from build123d import *

# Parameters (mm, degrees)
ESQUISSE2_W = 4
ESQUISSE2_H = 26
CONG_2_R    = 1
ESQUISSE3_W = 1.417366919
ESQUISSE3_H = 0.8


with BuildPart() as part:
    # Esquisse2 → Révolution1 (revolve)
    with BuildSketch(Plane.XY, mode=Mode.PRIVATE) as r_volution1_sk:
        with Locations((2, 13)):
            Rectangle(ESQUISSE2_W, ESQUISSE2_H)
    revolve(r_volution1_sk.sketch.rotate(Axis((0, 0, 0), (0, 1, 0)), 90), axis=Axis((0, 0, 0), (0, 1, 0)))

    # Congé2
    cong_2_edges = [part.edges().sort_by_distance(p)[0] for p in [
        (0, 0, 4),
        (0, 26, 4),
    ]]
    fillet(cong_2_edges, radius=CONG_2_R)

    # Esquisse3 → Enlèvement de matière-Révolution1 (revolve, cut)
    with BuildSketch(Plane.XY, mode=Mode.PRIVATE) as enl_vement_de_mati_re_r_volution1_sk:
        with Locations((-3.731857201, 21.6)):
            Rectangle(ESQUISSE3_W, ESQUISSE3_H)
    revolve(enl_vement_de_mati_re_r_volution1_sk.sketch.rotate(Axis((0, 0, 0), (0, -1, 0)), 270), axis=Axis((0, 0, 0), (0, -1, 0)), mode=Mode.SUBTRACT)


solid = part.part
For this review, take the finished solid that the model builds, in its own axes (mm). A direction names the side the tool comes from. Give positions to 0.01 mm unless a question says otherwise; leave off trailing zeros. Loops run counter-clockwise (first coordinate to the right, second up) from the corner with the lowest first, then second, coordinate; pieces in that order, holes last. Notation, with made-up numbers: (13.25, -9.75) -> (61.25, -9.75) arc R25 cw to (61.25, 29.25) -> close; hole circle Ø4 at (42.25, -32.5). An arc over 180 degrees is marked (long way). One line per question, with ' | ' between items.
1) Insertion check: pin 1 Ø4 at (x, y) = (-2.5, 4) entering from +Z; pin 2 Ø3 at (y, z) = (20, 2) entering from +X. Each pin has a flat end and moves straight along its axis. Give the tip position at first contact, or say it passes through.
Resolved:
pin 1: stops at z = 3.97 | pin 2: stops at x = 3.97
2) For faces 4 (the flat face through (-3, 22, -2)), 5 (the flat face through (0, 0, 0)), list the 3-axis set-ups (+Z, -Z, +X, -X, +Y, -Y) from which the entire face can be reached by the end or side of a thin tool; tool diameter is ignored.
Resolved:
face 4: none | face 5: +Z, -Z, +X, -X, -Y
3) The part is to be moulded in two halves that separate along Y. For faces 1 (the flat face through (0, 26, 0)), 2 (the cylindrical face through (3.905, 11.241, 0.867)), 3 (the cylindrical face through (2.68, 21.61, 1.4)), say which applies: +Y half, -Y half, draft (parallel to the pull), parting line (faces both ways), or undercut.
Resolved:
face 1: +Y half | face 2: draft | face 3: undercut
4) To check wall thickness, follow probe 1 along Y at (x, z) = (1.75, -3.5); probe 2 along X at (y, z) = (23.5, 0.75); probe 3 along Y at (x, z) = (-2.75, -2.75). State the ranges of each line that lie inside material, in increasing order.
Resolved:
probe 1: y = 0.59 to 21.2, 22 to 25.41 | probe 2: x = -3.93 to 3.93 | probe 3: y = 0.54 to 21.2, 22 to 25.46
5) We need section A-A (y = 22.5). Write out the cut boundary in (x, z).
Resolved:
outline: circle Ø8 at (0, 0)
